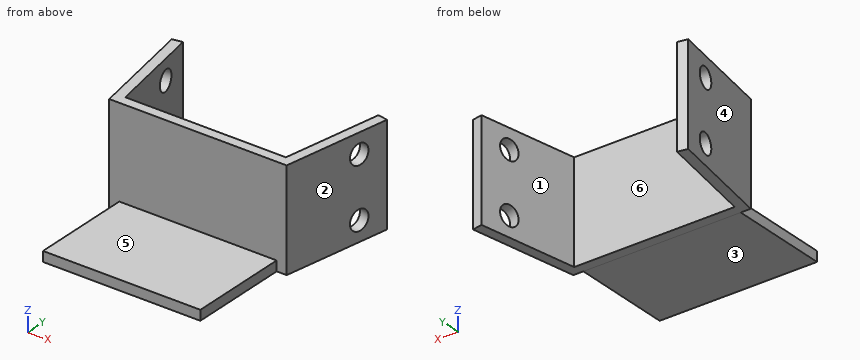
```python
from build123d import *

# Parameters (mm, degrees)
F1_DEPTH = 10
F2_R     = 1
F3_DEPTH = 1
F4_R     = 1
F5_DEPTH = 1
F7_DEPTH = 10


with BuildPart() as f1:
    # F0 (on Top) → F1 (new body)
    with BuildSketch(Plane.XY):
        Polygon((8, 0), (0, 0), (-8, 0), (-9.7364817767, 9.8480775301), (-10.7212895297, 9.6744293525), (-8.8390996312, -1), (0, -1), (8.8390996312, -1), (10.7212895297, 9.6744293525), (9.7364817767, 9.8480775301), align=None)
    extrude(amount=F1_DEPTH)

    # F2 (on face) → F3 (cut, through all)
    with BuildSketch(Plane(origin=(-8.7435782362, -1.541728751, 0), x_dir=(0.1736481777, -0.984807753, 0), z_dir=(-0.984807753, -0.1736481777, 0))):
        with Locations((-8.3891854213, 8)):
            Circle(F2_R)
        with Locations((-8.3891854213, 2)):
            Circle(F2_R)
    extrude(amount=-F3_DEPTH, mode=Mode.SUBTRACT)

    # F4 (on face) → F5 (cut, through all)
    with BuildSketch(Plane(origin=(8.7435782362, -1.541728751, 0), x_dir=(0.1736481777, 0.984807753, 0), z_dir=(0.984807753, -0.1736481777, 0))):
        with Locations((8.3891854213, 8)):
            Circle(F4_R)
        with Locations((8.3891854213, 2)):
            Circle(F4_R)
    extrude(amount=-F5_DEPTH, mode=Mode.SUBTRACT)

    # F6 (on face) → F7 (join)
    with BuildSketch(Plane.XZ.offset(1)):
        Polygon((7.8390996312, 1.3758e-06), (7.8390996312, 1.0000013758), (-7.8390996312, 0.9999986242), (-7.8390996312, -1.3758e-06), align=None)
    extrude(amount=F7_DEPTH)


solid = f1.part
```
Design review of the part built by this model. Coordinates are the model's own, in mm. Face numbers are marked on the shaded views. A direction names the side the tool comes from. Coordinates: 2 decimals unless noted, no trailing zeros. Write each loop counter-clockwise with the first axis right and the second up, starting at its lowest first coordinate (ties: lowest second). Pieces come first, ordered by that corner, then holes. Notation, with made-up numbers: M 1.25,62 L 12.25,62 A31 ccw 12.25,92 Z; hole C -32.5,43 d4. An arc over 180 degrees is marked long. Answer as a JSON object with one key per item and string values.
Item 1: Machinability: for the marked faces 4, 5 and 6, which of the approach directions +Z, -Z, +X, -X, +Y, -Y give a long, thin tool a straight path to every point of the face, cutting with its end or side? Answer none if there is none.
Outcome:
{"face 4": "+Z, -Z, -X, -Y", "face 5": "+Z, +X, -X, -Y", "face 6": "+Z, -Z, +Y"}
Item 2: Add section C-C, the plane y = 1.5. Give the boundary of the cut face in (x, z), and give its area (3 significant figures).
Outcome:
{"outline": "M -9.28,0 L -8.26,0 L -8.26,10 L -9.28,10 Z; M 8.26,0 L 9.28,0 L 9.28,10 L 8.26,10 Z", "area": "20.3 mm²"}
Item 3: Add section A-A, the plane x = -0.5. Give the boundary of the cut face in (y, z).
Outcome:
{"outline": "M -11,0 L 0,0 L 0,10 L -1,10 L -1,1 L -11,1 Z"}
Item 4: Draft analysis for pull direction X (two halves, no side actions). For the marked faces 1, 2 and 3, state which applies: pulls with the +X half, pulls with the -X half, needs draft (parallel to the pull), parting line crosses it, or undercut.
Outcome:
{"face 1": "undercut", "face 2": "pulls with the +X half", "face 3": "needs draft"}
Item 5: Insertion check: pin 1 Ø1.1 at (y, z) = (-4, 0.5) entering from -X; pin 2 Ø0.8 at (y, z) = (-7.5, 0.5) entering from +X; pin 3 Ø1.5 at (x, z) = (-7.5, 3) entering from -Y. Each pin has a flat end and moves straight along its axis. Give the tip position at first contact, or say it passes through.
Outcome:
{"pin 1": "x = -7.84", "pin 2": "x = 7.84", "pin 3": "y = -1"}
Item 6: Add section D-D, the plane z = 8.5. Give the boundary of the cut face in (x, y), and give its area (3 significant figures).
Outcome:
{"outline": "M -10.72,9.67 L -10.35,7.57 L -9.37,7.75 L -9.74,9.85 Z; M -10.05,5.87 L -8.84,-1 L 8.84,-1 L 10.05,5.87 L 9.07,6.04 L 8,0 L -8,0 L -9.07,6.04 Z; M 9.37,7.75 L 10.35,7.57 L 10.72,9.67 L 9.74,9.85 Z", "area": "34.2 mm²"}
Item 7: Add section B-B, the plane z = 5. Give the boundary of the cut face in (x, y).
Outcome:
{"outline": "M -10.72,9.67 L -8.84,-1 L 8.84,-1 L 10.72,9.67 L 9.74,9.85 L 8,0 L -8,0 L -9.74,9.85 Z"}
Item 8: Wall thickness on probe 1 along Y at (x, z) = (7.5, 2); probe 2 along Z at (x, y) = (4.75, -2.25); probe 3 along X at (y, z) = (6, 3.5): over which ranges is each line inside the solid? List them lowest first.
Outcome:
{"probe 1": "-1 to 0", "probe 2": "0 to 1", "probe 3": "-10.07 to -9.06, 9.06 to 10.07"}
